Verification items for the finished model (mm, model axes). Face numbers are marked on the shaded views. A direction names the side the tool comes from. Give positions to 0.01 mm unless a question says otherwise; leave off trailing zeros. Loops run counter-clockwise (first coordinate to the right, second up) from the corner with the lowest first, then second, coordinate; pieces in that order, holes last. Notation, with made-up numbers: M 64.25,-39 L 107.25,-39 A7 cw 107.25,-35 Z; hole C -39,-16.75 d2. An arc over 180 degrees is marked long. Use CSV: the item, a comma, the result in double quotes.
from build123d import *

# Parameters (mm, degrees)
F1_DEPTH = 25
F3_DEPTH = 70.001
F5_DEPTH = 2
F6_W     = 46
F6_H     = 19
F7_DEPTH = 20
F8_W     = 25
F8_H     = 19
F9_DEPTH = 66


with BuildPart() as f1:
    # F0 (on Top) → F1 (new body)
    with BuildSketch(Plane.XY):
        with BuildLine():
            Line((53.5, 0), (25, 0))
            ThreePointArc((25, 0), (7.32233, 7.32233), (0, 25))
            Line((0, 25), (0, 66))
            Line((0, 66), (-5, 66))
            Line((-5, 66), (-5, 46))
            Line((-5, 46), (-25, 0))
            Line((-25, 0), (-25, -4))
            Line((-25, -4), (120, -4))
            Line((120, -4), (120, 0))
            Line((120, 0), (113.5, 0))
            Line((113.5, 0), (112, 1.5))
            Line((112, 1.5), (110.5, 0))
            Line((110.5, 0), (109, 1.5))
            Line((109, 1.5), (107.5, 0))
            Line((107.5, 0), (106, 1.5))
            Line((106, 1.5), (104.5, 0))
            Line((104.5, 0), (103, 1.5))
            Line((103, 1.5), (101.5, 0))
            Line((101.5, 0), (100, 1.5))
            Line((100, 1.5), (98.5, 0))
            Line((98.5, 0), (97, 1.5))
            Line((97, 1.5), (95.5, 0))
            Line((95.5, 0), (94, 1.5))
            Line((94, 1.5), (92.5, 0))
            Line((92.5, 0), (91, 1.5))
            Line((91, 1.5), (89.5, 0))
            Line((89.5, 0), (88, 1.5))
            Line((88, 1.5), (86.5, 0))
            Line((86.5, 0), (85, 1.5))
            Line((85, 1.5), (83.5, 0))
            Line((83.5, 0), (82, 1.5))
            Line((82, 1.5), (80.5, 0))
            Line((80.5, 0), (79, 1.5))
            Line((79, 1.5), (77.5, 0))
            Line((77.5, 0), (76, 1.5))
            Line((76, 1.5), (74.5, 0))
            Line((74.5, 0), (73, 1.5))
            Line((73, 1.5), (71.5, 0))
            Line((71.5, 0), (70, 1.5))
            Line((70, 1.5), (68.5, 0))
            Line((68.5, 0), (67, 1.5))
            Line((67, 1.5), (65.5, 0))
            Line((65.5, 0), (64, 1.5))
            Line((64, 1.5), (62.5, 0))
            Line((62.5, 0), (61, 1.5))
            Line((61, 1.5), (59.5, 0))
            Line((59.5, 0), (58, 1.5))
            Line((58, 1.5), (56.5, 0))
            Line((56.5, 0), (55, 1.5))
            Line((55, 1.5), (53.5, 0))
        make_face()
    extrude(amount=F1_DEPTH)

    # F2 (on face) → F3 (cut, through all)
    with BuildSketch(Plane.XZ.offset(4)):
        with BuildLine():
            Line((60, 10.25), (110, 10.25))
            ThreePointArc((110, 10.25), (112.25, 12.5), (110, 14.75))
            Line((110, 14.75), (60, 14.75))
            ThreePointArc((60, 14.75), (57.75, 12.5), (60, 10.25))
        make_face()
    extrude(amount=-F3_DEPTH, mode=Mode.SUBTRACT)

    # F4 (on face) → F5 (cut)
    with BuildSketch(Plane.XZ.offset(4)):
        with BuildLine():
            Line((110, 17.75), (60, 17.75))
            ThreePointArc((60, 17.75), (54.75, 12.5), (60, 7.25))
            Line((60, 7.25), (110, 7.25))
            ThreePointArc((110, 7.25), (115.25, 12.5), (110, 17.75))
        make_face()
    extrude(amount=-F5_DEPTH, mode=Mode.SUBTRACT)

    # F6 (on face) → F7 (cut, through all)
    with BuildSketch(Plane(origin=(-25, 0, 0), x_dir=(0, -1, 0), z_dir=(-1, 0, 0))):
        with Locations((-23, 12.5)):
            Rectangle(F6_W, F6_H)
    extrude(amount=-F7_DEPTH, mode=Mode.SUBTRACT)

    # F8 (on face) → F9 (cut, through all)
    with BuildSketch(Plane(origin=(0, 66, 0), x_dir=(-1, 0, 0), z_dir=(0, 1, 0))):
        with Locations((-12.5, 12.5)):
            Rectangle(F8_W, F8_H)
    extrude(amount=-F9_DEPTH, mode=Mode.SUBTRACT)


solid = f1.part
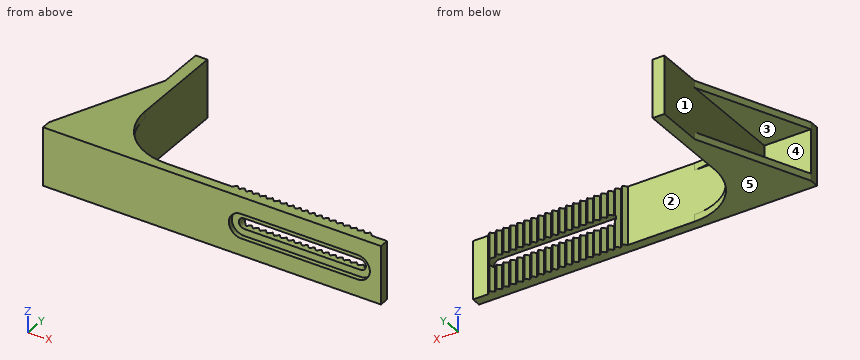
(1) Depth check by flat-ended pin: pin 1 Ø6 at (y, z) = (16, 11) entering from -X; pin 2 Ø7 at (x, z) = (116, 8) entering from +Y; pin 3 Ø1.5 at (x, z) = (74.5, 16.5) entering from +Y. Enter the tip coordinate at first touch or a pass-through.
Calculated:
pin 1,"stops at x = -5"
pin 2,"stops at y = 1"
pin 3,"stops at y = 0.75"
(2) Mould release check, pull along X, two halves, no side actions. Record for the marked faces 1, 2 and 3: released by +X, released by -X, zero draft, split by the parting line, or undercut.
Calculated:
face 1,"released by -X"
face 2,"undercut"
face 3,"zero draft"
(3) Scan lines: L1, parallel to Z at x = 1, y = 8.5; L2, parallel to Y at x = 32, z = 1.5; L3, parallel to X at y = 58.5, z = 3. Record each from-to range of solid material in increasing order. Write a range as from..to.
Calculated:
L1,"z = 0..3, 22..25"
L2,"y = -4..0"
L3,"x = -5..0"
(4) Section check A-A on x = 49. Record the cut outline in (y, z).
Calculated:
outline,"M -4,0 L 0,0 L 0,25 L -4,25 Z"
(5) Section check B-B on y = 51.5. Record the cut outline in (x, z).
Calculated:
outline,"M -5,0 L 0,0 L 0,25 L -5,25 Z"
(6) Tool access check on the marked faces 4 and 5. Record the directions out of +Z, -Z, +X, -X, +Y, -Y that give a thin tool (end or side, any length) a straight path to the whole face; none if there is none.
Calculated:
face 4,"-X, +Y"
face 5,"-Z, +X, -X, +Y, -Y"
